Autodesk Inventor part; units mm, degrees
ref_plane "YZ Plane" through (0, 0, 0) normal (1, 0, 0) x (0, 1, 0)
ref_plane "XZ Plane" through (0, 0, 0) normal (0, 1, 0) x (-1, 0, 0)
ref_plane "XY Plane" through (0, 0, 0) normal (0, 0, 1) x (1, 0, 0)
sketch "Sketch1" plane through (0, 0, 0) normal (0, 0, 1) x (1, 0, 0)
  line L0 (0, 0) -> (-530.225, 0)
  line L1 (-530.225, 0) -> (-530.225, -50.8)
  line L2 (-530.225, -50.8) -> (0, -50.8)
  line L3 (0, -50.8) -> (0, 0)
  line L4 (-403.225, 0) -> (-127, 0)
  line L5 (-127, 0) -> (-127, 50.8)
  line L6 (-127, 50.8) -> (-403.225, 50.8)
  line L7 (-403.225, 50.8) -> (-403.225, 0)
  line L8 (0, 50.8) -> (-530.225, 50.8)
  line L9 (-530.225, 50.8) -> (-530.225, 101.6)
  line L10 (-530.225, 101.6) -> (0, 101.6)
  line L11 (0, 101.6) -> (0, 50.8)
  line L12 (-530.225, 0) -> (-501.65, 0)
  line L13 (-501.65, 0) -> (-501.65, 50.8)
  line L14 (-501.65, 50.8) -> (-530.225, 50.8)
  line L15 (-530.225, 50.8) -> (-530.225, 0)
  line L16 (0, 0) -> (-28.575, 0)
  line L17 (-28.575, 0) -> (-28.575, 50.8)
  line L18 (-28.575, 50.8) -> (0, 50.8)
  line L19 (0, 50.8) -> (0, 0)
  dimension "d0" = 530.225
  dimension "d1" = 50.8
  dimension "d2" = 50.8
  dimension "d3" = 127
  dimension "d4" = 127
  dimension "d5" = 50.8
  dimension "d6" = 530.225
  dimension "d7" = 0
  dimension "d8" = 50.8
  dimension "d9" = 28.575
  dimension "d10" = 28.575
extrude "Extrusion1" add sketch "Sketch1" along normal blind 3.175 contours L3 L2 L1 L0 | L0 L17 L8 L19 | L8 L6 L9 L10 L11 | L0 L7 L6 L5 | L15 L8 L13 L0
sketch "Sketch2" plane through (0, 0, 3.175) normal (0, 0, 1) x (1, 0, 0)
  line L0 (-352.425, 63.5) -> (-177.8, 63.5) construction
  line L1 (-177.8, 63.5) -> (-177.8, -1.2974) construction
  line L2 (-177.8, -1.2974) -> (-352.425, -1.2974) construction
  line L3 (-352.425, -1.2974) -> (-352.425, 63.5) construction
  line L4 (-403.225, 50.8) -> (-403.225, 0)
  line L5 (-127, 0) -> (-127, 50.8)
  line L6 (0, 101.6) -> (-530.225, 101.6)
  spline S0 degree 2 poles (-311.0058, -6.6857) (-311.0058, -12.7) (-317.0201, -12.7) knots 0 0 0 1 1 1
  line L7 (-317.0201, -12.7) -> (-341.8149, -12.7)
  spline S1 degree 2 poles (-341.8149, -12.7) (-347.8292, -12.7) (-347.8292, -6.6857) knots 0 0 0 1 1 1
  line L8 (-347.8292, -6.6857) -> (-347.8292, 57.4857)
  spline S2 degree 2 poles (-347.8292, 57.4857) (-347.8292, 63.5) (-341.9284, 63.5) knots 0 0 0 1 1 1
  line L9 (-341.9284, 63.5) -> (-317.247, 63.5)
  spline S3 degree 2 poles (-317.247, 63.5) (-311.176, 63.5) (-311.176, 57.4857) knots 0 0 0 1 1 1
  line L10 (-311.176, 57.4857) -> (-311.176, 40.4074)
  line L11 (-311.176, 40.4074) -> (-322.3535, 40.4074)
  line L12 (-322.3535, 40.4074) -> (-322.3535, 53.741)
  line L13 (-322.3535, 53.741) -> (-336.6517, 53.741)
  line L14 (-336.6517, 53.741) -> (-336.6517, 30.8185)
  line L15 (-336.6517, 30.8185) -> (-317.0201, 30.8185)
  spline S4 degree 2 poles (-317.0201, 30.8185) (-311.0058, 30.8185) (-311.0058, 24.8042) knots 0 0 0 1 1 1
  line L16 (-311.0058, 24.8042) -> (-311.0058, -6.6857)
  line L17 (-322.1266, -2.941) -> (-322.1266, 21.1162)
  line L18 (-322.1266, 21.1162) -> (-336.6517, 21.1162)
  line L19 (-336.6517, 21.1162) -> (-336.6517, -2.941)
  line L20 (-336.6517, -2.941) -> (-322.1266, -2.941)
  spline S5 degree 2 poles (-265.161, -6.6857) (-265.161, -12.7) (-271.1753, -12.7) knots 0 0 0 1 1 1
  line L21 (-271.1753, -12.7) -> (-296.0835, -12.7)
  spline S6 degree 2 poles (-296.0835, -12.7) (-301.8141, -12.7) (-301.8141, -6.6857) knots 0 0 0 1 1 1
  line L22 (-301.8141, -6.6857) -> (-301.8141, 10.3926)
  line L23 (-301.8141, 10.3926) -> (-290.6366, 10.3926)
  line L24 (-290.6366, 10.3926) -> (-290.6366, -2.941)
  line L25 (-290.6366, -2.941) -> (-276.452, -2.941)
  line L26 (-276.452, -2.941) -> (-276.452, 19.9815)
  line L27 (-276.452, 19.9815) -> (-296.4807, 19.9815)
  spline S7 degree 2 poles (-296.4807, 19.9815) (-302.0978, 19.9815) (-302.0978, 25.9958) knots 0 0 0 1 1 1
  line L28 (-302.0978, 25.9958) -> (-302.0978, 57.4857)
  spline S8 degree 2 poles (-302.0978, 57.4857) (-302.0978, 63.5) (-296.4807, 63.5) knots 0 0 0 1 1 1
  line L29 (-296.4807, 63.5) -> (-271.2887, 63.5)
  spline S9 degree 2 poles (-271.2887, 63.5) (-265.161, 63.5) (-265.161, 57.4857) knots 0 0 0 1 1 1
  line L30 (-265.161, 57.4857) -> (-265.161, -6.6857)
  line L31 (-276.452, 29.627) -> (-276.452, 53.741)
  line L32 (-276.452, 53.741) -> (-290.977, 53.741)
  line L33 (-290.977, 53.741) -> (-290.977, 29.627)
  line L34 (-290.977, 29.627) -> (-276.452, 29.627)
  spline S10 degree 2 poles (-218.3516, -6.6857) (-218.3516, -12.7) (-224.3659, -12.7) knots 0 0 0 1 1 1
  line L35 (-224.3659, -12.7) -> (-250.0117, -12.7)
  spline S11 degree 2 poles (-250.0117, -12.7) (-256.026, -12.7) (-256.026, -6.6857) knots 0 0 0 1 1 1
  line L36 (-256.026, -6.6857) -> (-256.026, 16.4069)
  spline S12 degree 2 poles (-256.026, 16.4069) (-256.026, 20.6056) (-253.1891, 22.8751) knots 0 0 0 1 1 1
  spline S13 degree 2 poles (-253.1891, 22.8751) (-249.8415, 24.8042) (-246.4372, 26.7901) knots 0 0 0 1 1 1
  spline S14 degree 2 poles (-246.4372, 26.7901) (-249.7281, 28.6625) (-252.9622, 30.5916) knots 0 0 0 1 1 1
  spline S15 degree 2 poles (-252.9622, 30.5916) (-255.9126, 32.9179) (-255.9126, 36.8896) knots 0 0 0 1 1 1
  line L37 (-255.9126, 36.8896) -> (-255.9126, 57.4857)
  spline S16 degree 2 poles (-255.9126, 57.4857) (-255.9126, 63.5) (-249.7281, 63.5) knots 0 0 0 1 1 1
  line L38 (-249.7281, 63.5) -> (-224.4794, 63.5)
  spline S17 degree 2 poles (-224.4794, 63.5) (-218.5218, 63.5) (-218.5218, 57.4857) knots 0 0 0 1 1 1
  line L39 (-218.5218, 57.4857) -> (-218.5218, 36.8896)
  spline S18 degree 2 poles (-218.5218, 36.8896) (-218.5218, 32.8611) (-221.4722, 30.5916) knots 0 0 0 1 1 1
  spline S19 degree 2 poles (-221.4722, 30.5916) (-224.7063, 28.6625) (-227.9972, 26.7901) knots 0 0 0 1 1 1
  spline S20 degree 2 poles (-227.9972, 26.7901) (-224.6496, 24.8042) (-221.2453, 22.8751) knots 0 0 0 1 1 1
  spline S21 degree 2 poles (-221.2453, 22.8751) (-218.3516, 20.6056) (-218.3516, 16.4069) knots 0 0 0 1 1 1
  line L40 (-218.3516, 16.4069) -> (-218.3516, -6.6857)
  line L41 (-229.6993, -3.1112) -> (-229.6993, 17.9956)
  line L42 (-229.6993, 17.9956) -> (-237.1888, 22.3077)
  line L43 (-237.1888, 22.3077) -> (-244.7351, 17.9956)
  line L44 (-244.7351, 17.9956) -> (-244.7351, -3.1112)
  line L45 (-244.7351, -3.1112) -> (-229.6993, -3.1112)
  line L46 (-229.8128, 35.6413) -> (-229.8128, 53.9112)
  line L47 (-229.8128, 53.9112) -> (-244.5648, 53.9112)
  line L48 (-244.5648, 53.9112) -> (-244.5648, 35.6413)
  line L49 (-244.5648, 35.6413) -> (-237.1888, 31.2725)
  line L50 (-237.1888, 31.2725) -> (-229.8128, 35.6413)
  point P0 (0, 0)
  dimension "d13" = 50.8
  dimension "d14" = 50.8
  dimension "d15" = 38.1
extrude "Extrusion2" cut sketch "Sketch2" against normal blind 0.7937
sketch "Sketch3" plane through (0, 0, 3.175) normal (0, 0, 1) x (1, 0, 0)
  point P0 (0, 0)
properties part number "upper Ramp"
Work out the finished part from the listing and answer in its coordinate system (mm). Coordinates: 2 decimals unless noted, no trailing zeros. Write each loop counter-clockwise with the first axis right and the second up, starting at its lowest first coordinate (ties: lowest second). Pieces come first, ordered by that corner, then holes.
1. A flat-ended cylindrical pin translates along its axis: pin 1 (5 mm diameter, centred on x = -315, y = -8.5, fed in from +Z). Find the tip coordinate at first contact, or state that the pin passes through.
Results list:
pin 1: stops at z = 2.38
2. Consider line 1 along X through (y, z) = (33.5, 0.75) (3 decimals); line 2 along Y through (x, z) = (-39.5, 2.2); line 3 along Z through (x, y) = (-292.5, 59.5). Determine where each line is inside the solid, lowest interval first.
Results list:
line 1: x = -530.225 to -501.65, -403.225 to -127, -28.575 to 0
line 2: y = -50.8 to 0, 50.8 to 101.6
line 3: z = 0 to 2.38
3. The part is cut by section B-B, the plane z = 1.5. Write down the section's boundary in (x, y) (3 decimals), and give its area (3 significant figures).
Results list:
outline: (-530.225, -50.8) - (0, -50.8) - (0, 101.6) - (-530.225, 101.6) - close; hole (-501.65, 0) - (-403.225, 0) - (-403.225, 50.8) - (-501.65, 50.8) - close; hole (-127, 0) - (-28.575, 0) - (-28.575, 50.8) - (-127, 50.8) - close
area: 70,800 mm2
4. The part is cut by section A-A, the plane x = -51. Write down the section's boundary in (y, z) (3 decimals), and give its area (3 significant figures).
Results list:
outline: (-50.8, 0) - (0, 0) - (0, 3.175) - (-50.8, 3.175) - close; (50.8, 0) - (101.6, 0) - (101.6, 3.175) - (50.8, 3.175) - close
area: 323 mm2
5. For a pull along Y with two mould halves and no side action, classify faces 1 (the flat face through (-330, 26, 2.381)), 2 (the flat face through (-237, 43, 3.175)) as +Y half, -Y half, draft (parallel to the pull), parting line (faces both ways), or undercut.
Results list:
face 1: undercut
face 2: draft
